CAD build for the part. Positions are in the model's coordinates, mm. A direction names the side the tool comes from. Coordinates: 2 decimals unless noted, no trailing zeros. Loops run counter-clockwise (first coordinate to the right, second up) from the corner with the lowest first, then second, coordinate; pieces in that order, holes last. Notation, with made-up numbers: (82.25, -28) -> (92.25, -28) arc R31 ccw to (92.25, 2) -> close; hole circle Ø5 at (35.25, 41). An arc over 180 degrees is marked (long way). Write each question's results on one line, items separated by ' | '.
```python
from build123d import *

# Parameters (mm, degrees)
F1_DEPTH = 5
F2_W     = 110
F2_H     = 110
F3_DEPTH = 2.5
F4_W     = 110
F4_H     = 110
F5_DEPTH = 2.5


with BuildPart() as f1:
    # F0 (on Front) → F1 (new body)
    with BuildSketch(Plane.XZ):
        Polygon((51.25, -29.589201), (0, 59.178403), (-51.25, -29.589201), align=None)
    extrude(amount=-F1_DEPTH)

    # F2 (on face) → F3 (join, symmetric)
    with BuildSketch(Plane(origin=(-25.625, 0, 14.794601), x_dir=(0, -1, 0), z_dir=(-0.866025, 0, 0.5))):
        with Locations((50, -3.75)):
            Rectangle(F2_W, F2_H)
    extrude(amount=F3_DEPTH, both=True)

    # F4 (on face) → F5 (join, symmetric)
    with BuildSketch(Plane(origin=(25.625, 0, 14.794601), x_dir=(0, 1, 0), z_dir=(0.866025, 0, 0.5))):
        with Locations((-50, -5.915064)):
            Rectangle(F4_W, F4_H)
    extrude(amount=F5_DEPTH, both=True)


solid = f1.part
```
Q1. Cut at D-D on x = -22. Write the cut outline in (y, z).
Results are:
outline: (-105, 16.07) -> (0, 16.07) -> (0, -29.59) -> (5, -29.59) -> (5, 26.07) -> (-105, 26.07) -> close
Q2. Cut at C-C on x = -35. Write the cut outline in (y, z), and give its area (3 significant figures).
Results are:
outline: (-105, -6.44) -> (0, -6.44) -> (0, -29.59) -> (5, -29.59) -> (5, 3.56) -> (-105, 3.56) -> close | area: 1,220 mm^2
Q3. Pull direction X, two halves, no side cores. Call faces 1 (the flat face through (-20, -105, 23)), 2 (the flat face through (-55.03, -49.23, -36.067)), 3 (the flat face through (-26.05, -49.23, 9.06)), 4 (the flat face through (26.58, -50.77, 8.14)): +X half, -X half, draft (parallel to the pull), parting line (faces both ways), or undercut.
Results are:
face 1: draft | face 2: -X half | face 3: undercut | face 4: undercut
Q4. Cut at A-A on y = -42.5. Write the cut outline in (x, z).
Results are:
outline: (-57.17, -34.83) -> (-52.83, -37.33) -> (0, 54.18) -> (53.92, -39.21) -> (58.25, -36.71) -> (3.25, 58.55) -> (2.17, 57.93) -> (-2.17, 60.43) -> close
Q5. Cut at B-B on z = 10. Write the cut outline in (x, y).
Results are:
outline: (-31.28, -105) -> (-25.51, -105) -> (-25.51, 0) -> (25.51, 0) -> (25.51, -105) -> (31.28, -105) -> (31.28, 5) -> (-31.28, 5) -> close
Q6. Drop flat-ended pins along their axis: pin 1 (2 mm diameter, centred on y = -27.5, z = 14.5, fed in from +X); pin 2 (1 mm diameter, centred on x = 34.5, z = -19, fed in from -Y); pin 3 (6 mm diameter, centred on y = -61.5, z = -6.5, fed in from -X). Give the stop position or say it passes through.
Results are:
pin 1: x = 29.26 | pin 2: y = 0 | pin 3: x = -42.54
Q7. Which spindle directions (+Z, -Z, +X, -X, +Y, -Y) get a long thin tool onto all of the face, cutting with end or side? Do faces 5 (the flat face through (56.113, -50.77, -37.942)), 6 (the flat face through (7, 5, -1)), 7 (the flat face through (-1, 2, -29.589)), 8 (the flat face through (-0.03, -49.23, 59.196)), 9 (the flat face through (-1, 0, 4)). Say none if no direction does.
Results are:
face 5: -Z, +X, +Y, -Y | face 6: +Z, -Z, +X, -X, +Y | face 7: -Z, +Y, -Y | face 8: +Z, +Y, -Y | face 9: -Z, -Y
Q8. Wall check: L1, parallel to Y at x = 9, z = -27; L2, parallel to X at y = -1, z = 38; L3, parallel to X at y = -94, z = 4.5. Give the ranges that are in metal, low to high. Write a range as from..to.
Results are:
L1: 0..5 | L2: -15.11..-9.34, 9.34..15.11 | L3: -34.46..-28.68, 28.68..34.46
